Autodesk Inventor part; units mm, degrees
ref_plane "YZ Plane" through (0, 0, 0) normal (1, 0, 0) x (0, 1, 0)
ref_plane "XZ Plane" through (0, 0, 0) normal (0, 1, 0) x (-1, 0, 0)
ref_plane "XY Plane" through (0, 0, 0) normal (0, 0, 1) x (1, 0, 0)
sketch "Sketch1" plane through (0, 0, 0) normal (0, 1, 0) x (-1, 0, 0)
  line L0 (0, 0) -> (-70, 0)
  line L1 (-70, 0) -> (-70, 165)
  line L2 (-70, 165) -> (0, 165)
  line L3 (0, 165) -> (0, 0)
  dimension "d0" = 70
  dimension "d1" = 165
extrude "Extrusion1" add sketch "Sketch1" along normal blind 7
sketch "Sketch2" plane through (0, 0, 0) normal (0, -1, 0) x (1, 0, 0)
  line L0 (70, 165) -> (70, 0)
  line L1 (70, 0) -> (55, 0)
  line L2 (55, 0) -> (55, 15.9792)
  line L3 (55, 15.9792) -> (70, 15.9792)
  line L4 (70, 15.9792) -> (70, 0)
  line L5 (70, 0) -> (0, 0)
  line L6 (0, 0) -> (15, 0)
  line L7 (15, 0) -> (15, 13.5714)
  line L8 (15, 13.5714) -> (0, 13.5714)
  line L9 (0, 13.5714) -> (0, 0)
  line L10 (70, 165.2646) -> (55, 165.2646)
  line L11 (55, 165.2646) -> (55, 149.7232)
  line L12 (55, 149.7232) -> (70, 149.7232)
  line L13 (70, 149.7232) -> (70, 165.2646)
  line L14 (0, 165.2646) -> (15, 165.2646)
  line L15 (15, 165.2646) -> (15, 148.1909)
  line L16 (15, 148.1909) -> (0, 148.1909)
  line L17 (0, 148.1909) -> (0, 165.2646)
  line L18 (68, 151.7232) -> (57, 151.7232)
  line L19 (57, 151.7232) -> (57, 163.2646)
  line L20 (57, 163.2646) -> (68, 163.2646)
  line L21 (68, 163.2646) -> (68, 151.7232)
  line L22 (2, 150.1909) -> (13, 150.1909)
  line L23 (13, 150.1909) -> (13, 163.2646)
  line L24 (13, 163.2646) -> (2, 163.2646)
  line L25 (2, 163.2646) -> (2, 150.1909)
  line L26 (2, 11.5714) -> (13, 11.5714)
  line L27 (13, 11.5714) -> (13, 2)
  line L28 (13, 2) -> (2, 2)
  line L29 (2, 2) -> (2, 11.5714)
  line L30 (68, 13.9792) -> (57, 13.9792)
  line L31 (57, 13.9792) -> (57, 2)
  line L32 (57, 2) -> (68, 2)
  line L33 (68, 2) -> (68, 13.9792)
  dimension "d4" = 15
  dimension "d5" = 15
  dimension "d6" = 15
  dimension "d7" = 15
  dimension "d8" = 2
  dimension "d9" = 2
  dimension "d10" = 2
  dimension "d11" = 2
extrude "Extrusion2" add sketch "Sketch2" along normal blind 41
sketch "Sketch3" plane through (0, 7, 0) normal (0, 1, 0) x (1, 0, 0)
  line L0 (18.4911, -158.4869) -> (54.4911, -158.4869) construction
  line L1 (0, -165) -> (70, -165)
  line L2 (0, -165) -> (0, -129)
  line L3 (0, -13.5714) -> (0, -148.1909)
  line L4 (0, -129) -> (70, -129)
  line L5 (70, -165) -> (70, 0)
  line L6 (70, -129) -> (5, -129)
  line L7 (5, -129) -> (5, -120.5)
  line L8 (5, -120.5) -> (70, -120.5)
  line L9 (70, -120.5) -> (70, -129)
  line L10 (70, -110.5) -> (5, -110.5)
  line L11 (5, -110.5) -> (5, -102)
  line L12 (5, -102) -> (70, -102)
  line L13 (70, -102) -> (70, -110.5)
  line L14 (5, -102) -> (65, -102)
  line L15 (65, -182) -> (5, -182)
  line L16 (5, -182) -> (5, -102)
  line L17 (5, -120.5) -> (65, -120.5)
  line L18 (65, -120.5) -> (65, -129)
  line L19 (65, -129) -> (5, -129)
  line L20 (5, -129) -> (5, -120.5)
  line L21 (5, -102) -> (65, -102)
  line L22 (65, -102) -> (65, -110.5)
  line L23 (65, -110.5) -> (5, -110.5)
  line L24 (5, -110.5) -> (5, -102)
  point P0 (0, 0)
  dimension "d16" = 36
  dimension "d17" = 65
  dimension "d18" = 8.5
  dimension "d20" = 65
  dimension "d21" = 8.5
  dimension "d22" = 60
  dimension "d23" = 80
  dimension "d24" = 60
  dimension "d25" = 8.5
  dimension "d26" = 60
  dimension "d27" = 8.5
extrude "Extrusion3" cut sketch "Sketch3" against normal blind 7 contours L7 L8 L18 L4 | L11 L12 L22 L10
sketch "Sketch4" plane through (0, 7, 0) normal (0, 1, 0) x (1, 0, 0)
  line L0 (35, -52.8248) -> (30, -52.8248)
  line L1 (30, -52.8248) -> (30, -81.8248)
  line L2 (30, -81.8248) -> (35, -81.8248)
  line L3 (35, -81.8248) -> (35, -52.8248)
  line L4 (37, -50.8248) -> (28, -50.8248)
  line L5 (28, -50.8248) -> (28, -83.8248)
  line L6 (28, -83.8248) -> (37, -83.8248)
  line L7 (37, -83.8248) -> (37, -50.8248)
  point P0 (0, 0)
  dimension "d30" = 5
  dimension "d31" = 29
  dimension "d32" = 2
extrude "Extrusion4" add sketch "Sketch4" along normal blind 29
sketch "Sketch5" plane through (28, 7, 50.8248) normal (-1, 0, 0) x (0, 0, 1)
  line L0 (2, 0) -> (2, 29)
  line L1 (2, 29) -> (2, 0)
  line L2 (31, 0) -> (31, 29)
  line L3 (2, 0) -> (31, 0)
  line L4 (31, 0) -> (31, 29)
  line L5 (31, 29) -> (2, 29)
  line L6 (2, 29) -> (31, 29)
  line L7 (31, 29) -> (31, 26)
  line L8 (31, 26) -> (2, 26)
  line L9 (2, 26) -> (2, 29)
  line L10 (2, 26) -> (31, 26)
  line L11 (31, 26) -> (31, 0)
  line L12 (31, 0) -> (2, 0)
  line L13 (2, 0) -> (2, 26)
  point P0 (-50.8248, -7)
  dimension "d35" = 29
  dimension "d36" = 3
extrude "Extrusion5" cut sketch "Sketch5" against normal blind 2 contours L0 L8 L2 L3
sketch "Sketch6" plane through (37, 7, 83.8248) normal (1, 0, 0) x (0, 0, -1)
  line L0 (2, 29) -> (31, 29)
  line L1 (16.5, 29) -> (16.5, 0)
  line L2 (2, 0) -> (31, 0)
  line L3 (23.5, 29) -> (23.5, 0)
  line L4 (9.5, 29) -> (9.5, 0)
  line L5 (9.5, 29) -> (23.5, 29)
  line L6 (23.5, 29) -> (23.5, 0)
  line L7 (23.5, 0) -> (9.5, 0)
  line L8 (9.5, 0) -> (9.5, 29)
  point P0 (83.8248, -7)
  point P1 (23.5, 0)
  point P2 (23.5, 29)
  point P3 (9.5, 29)
  point P4 (9.5, 0)
  dimension "d39" = 7
  dimension "d40" = 7
extrude "Extrusion6" cut sketch "Sketch6" against normal blind 2
sketch "Sketch7" plane through (28, 33, 52.8248) normal (0, -1, 0) x (1, 0, 0)
  line L0 (0, 0) -> (0, 29)
  line L1 (2, 29) -> (2, 0)
  line L2 (0, 0) -> (2, 0)
  line L3 (2, 0) -> (2, 29)
  line L4 (2, 29) -> (0, 29)
  line L5 (0, 29) -> (0, 0)
  point P0 (-28, -52.8248)
  point P1 (2, 0)
extrude "Extrusion7" add sketch "Sketch7" along normal blind 2
properties part number "piano laterale"
Input: part model. Units: mm. Frame: model coordinates. A direction names the side the tool comes from. Give positions to 0.01 mm unless a question says otherwise; leave off trailing zeros. Loops run counter-clockwise (first coordinate to the right, second up) from the corner with the lowest first, then second, coordinate; pieces in that order, holes last. Notation, with made-up numbers: M -37,82 L 2,82 A15 ccw 2,107 Z; hole C 87,1 d5. An arc over 180 degrees is marked long. Answer as CSV lines item,"result". Start each with the question number.
1. Section A-A on z = 76. Return loops of the section in (x, y).
2. Section C-C on x = 45. Return loops of the section in (y, z).
3. Line query: L1, parallel to Z at x = 16, y = 6; L2, parallel to Z at x = 66, y = -11.5; L3, parallel to Z at x = 29, y = 30. Output: solid intervals per line, ascending.
4. Section D-D on y = -25.5. State how many separate pieces and enclosed holes the cut face has, plus the area to 3 significant figures.
5. Pin query (flat end, axial travel): P1, Ø8, axis at x = 12, z = 137.5, coming from the +Y side; P2, Ø1.5, axis at x = 34.5, z = 32, coming from the -Y side; P3, Ø6, axis at x = 38, y = 23, coming from the -Z side. Return the tip coordinate at first contact, or that it passes through.
6. Section B-B on y = 22.5. Return loops of the section in (x, z), plus the area to 3 significant figures.
7. Reachability of faces 1 (the face through (35, 4, 120.5)), 2 (the face through (8, -20, 163.265)), 3 (the face through (15, -20, 157)), 4 (the face through (35, 3, 165)) from +Z, -Z, +X, -X, +Y, -Y: full face, straight path, thin tool, end or side. Return the list, or none.
8. Pull-direction query (Y, two-part tool) for faces 5 (the face through (69, -41, 158)), 6 (the face through (31, 21, 52.825)), 7 (the face through (33, 21, 50.825)); classes: released by +Y, released by -Y, zero draft, split by the parting line, or undercut.
Computed values:
1,outline,"M 0,0 L 70,0 L 70,7 L 37,7 L 37,36 L 35,36 L 35,7 L 0,7 Z; M 28,31 L 30,31 L 30,36 L 28,36 Z"
2,outline,"M 0,0 L 7,0 L 7,102 L 0,102 Z; M 0,110.5 L 7,110.5 L 7,120.5 L 0,120.5 Z; M 0,129 L 7,129 L 7,165 L 0,165 Z"
3,L1,"z = 0 to 102, 110.5 to 120.5, 129 to 165"
3,L2,"z = 0 to 2, 13.98 to 15.98, 149.72 to 151.72, 163.26 to 165.26"
3,L3,"z = 50.82 to 52.82, 81.82 to 83.82"
4,separate pieces,"4"
4,enclosed holes,"4"
4,area,"425 mm²"
5,P1,"stops at y = 7"
5,P2,"stops at y = 0"
5,P3,"stops at z = 50.82"
6,outline,"M 28,50.82 L 37,50.82 L 37,60.32 L 35,60.32 L 35,52.82 L 28,52.82 Z; M 28,81.82 L 35,81.82 L 35,74.32 L 37,74.32 L 37,83.82 L 28,83.82 Z"
6,area,"66.0 mm²"
7,face 1,"+Y, -Y"
7,face 2,"-Y"
7,face 3,"+Z, -Z, -Y"
7,face 4,"+Z, +X, -X, +Y"
8,face 5,"released by -Y"
8,face 6,"undercut"
8,face 7,"zero draft"
